from build123d import *

# Parameters (mm, degrees)
SKETCH_1_R          = 4.5
EXTRUDE_1_DEPTH     = 5
CUT_EXTRUDE_1_DEPTH = 10


with BuildPart() as part:
    # 草图1 → 凸台-拉伸1 (new body)
    with BuildSketch(Plane(origin=(0, 0, 0), x_dir=(1, 0, 0), z_dir=(0, 1, 0))):
        with BuildLine():
            Line((-39.403034963, -93.411939556), (2.365895093, -108.411939556))
            ThreePointArc((2.365895093, -108.411939556), (6.588060444, -117.365895093), (-2.365895093, -121.588060444))
            Line((-2.365895093, -121.588060444), (-44.134825149, -106.588060444))
            ThreePointArc((-44.134825149, -106.588060444), (-48.356990499, -97.634104907), (-39.403034963, -93.411939556))
        make_face()
        with Locations(Location((-41.768930056, -100, 0), (0, 0, 270))):
            Circle(SKETCH_1_R, mode=Mode.SUBTRACT)
        with Locations(Location((0, -115, 0), (0, 0, 270))):
            Circle(SKETCH_1_R, mode=Mode.SUBTRACT)
    extrude(amount=EXTRUDE_1_DEPTH)

    # 草图2 → 切除-拉伸1 (cut)
    with BuildSketch(Plane(origin=(0, 5, 0), x_dir=(1, 0, 0), z_dir=(0, 1, 0))):
        with BuildLine():
            Line((-30.561161413, -101.89986187), (-9.85582859, -109.335532162))
            ThreePointArc((-9.85582859, -109.335532162), (-8.649495632, -111.893805173), (-11.207768643, -113.10013813))
            Line((-11.207768643, -113.10013813), (-31.913101466, -105.664467838))
            ThreePointArc((-31.913101466, -105.664467838), (-33.119434423, -103.106194827), (-30.561161413, -101.89986187))
        make_face()
    extrude(amount=-CUT_EXTRUDE_1_DEPTH, mode=Mode.SUBTRACT)


solid = part.part
Check sheet for the modelled part. Datum: model origin and axes. Units: mm. A direction names the side the tool comes from. Coordinates: 2 decimals unless noted, no trailing zeros. Loops run counter-clockwise (first coordinate to the right, second up) from the corner with the lowest first, then second, coordinate; pieces in that order, holes last. Notation, with made-up numbers: (0.25, 75) -> (19.25, 75) arc R10 ccw to (19.25, 79) -> close; hole circle Ø4 at (6, -14). An arc over 180 degrees is marked (long way). Answer in a Markdown table with one row per item.
1. Sectioned sample at C-C, the plane x = 0. Record the boundary of the cut face in (y, z), then the cut area to 3 significant figures.
Check values:
| item | result |
|---|---|
| outline | (0, 107.56) -> (5, 107.56) -> (5, 110.5) -> (0, 110.5) -> close; (0, 119.5) -> (5, 119.5) -> (5, 122) -> (0, 122) -> close |
| area | 27.2 mm2 |
2. Go/stop test with flat-tipped pins: pin 1 (5.5 mm diameter, centred on x = -41.77, z = 100, fed in from -Y); pin 2 (1 mm diameter, centred on x = -40.5, y = 2.5, fed in from -Z); pin 3 (1 mm diameter, centred on y = 3.5, z = 118, fed in from +X); pin 4 (3 mm diameter, centred on x = -23, y = 3.5, fed in from +Z). Record where each tip stops, or that it passes through.
Check values:
| item | result |
|---|---|
| pin 1 | passes through |
| pin 2 | stops at z = 93.04 |
| pin 3 | stops at x = 6.54 |
| pin 4 | stops at z = 114.72 |
3. Release check for a two-part mould opening along Z. For faces 1 (the face through (-21, 0, 105)), 2 (the face through (-20.353, 2.535, 105.566)), 3 (the face through (-22.958, 2.465, 114.193)), 4 (the face through (-48.407, 2.465, 97.78)) record: released by +Z, released by -Z, zero draft, split by the parting line, or undercut.
Check values:
| item | result |
|---|---|
| face 1 | zero draft |
| face 2 | undercut |
| face 3 | released by +Z |
| face 4 | split by the parting line |
4. Material ranges on line 1 along Z through (x, y) = (0.5, 1.15); line 2 along Z through (x, y) = (-45.5, 0.55); line 3 along Z through (x, y) = (-36, 3.2), recorded low to high. Write a range as [from, to].
Check values:
| item | result |
|---|---|
| line 1 | z = [107.74, 110.53], [119.47, 121.98] |
| line 2 | z = [94.08, 97.48], [102.52, 105.92] |
| line 3 | z = [94.63, 109.51] |
5. Sectioned sample at A-A, the plane z = 97. Record the boundary of the cut face in (x, y), then the cut area to 3 significant figures.
Check values:
| item | result |
|---|---|
| outline | (-48.09, 0) -> (-45.12, 0) -> (-45.12, 5) -> (-48.09, 5) -> close; (-38.41, 0) -> (-29.41, 0) -> (-29.41, 5) -> (-38.41, 5) -> close |
| area | 59.9 mm2 |
6. Access from +Z, -Z, +X, -X, +Y, -Y to the whole of each face (thin tool, end or side, straight path). Record for faces 5 (the face through (-21.415, 2.535, 109.434)), 6 (the face through (-21, 5, 105)).
Check values:
| item | result |
|---|---|
| face 5 | +Y, -Y |
| face 6 | +Z, -Z, +X, -X, +Y |
7. Sectioned sample at B-B, the plane y = 4.25. Record the boundary of the cut face in (x, z).
Check values:
| item | result |
|---|---|
| outline | (-44.13, 106.59) arc R7 ccw to (-39.4, 93.41) -> (2.37, 108.41) arc R7 ccw to (-2.37, 121.59) -> close; hole circle Ø9 at (-41.77, 100); hole (-31.91, 105.66) arc R2 ccw to (-30.56, 101.9) -> (-9.86, 109.34) arc R2 ccw to (-11.21, 113.1) -> close; hole circle Ø9 at (0, 115) |
